Source: CAD feature listing. Evaluate the final solid. Frame: model axes, mm. Give positions to 0.01 mm unless a question says otherwise; leave off trailing zeros. Order: outer loops, then holes, each group sorted by start corner. A loop starts at its lowest first (then second) coordinate and runs counter-clockwise, first axis right, second up. Notation, with made-up numbers: M 36,7.5 L 63,7.5 A10 cw 63,24.5 Z; hole C -7,45 d7. An arc over 180 degrees is marked long. Return JSON: item names as keys, results as strings.
from build123d import *

# Parameters (mm, degrees)
F0_W     = 57.15
F0_H     = 38.1
F1_DEPTH = 25.4
F3_DEPTH = 25.4
F5_DEPTH = 25.4


with BuildPart() as f1:
    # F0 (on Front) → F1 (new body)
    with BuildSketch(Plane.XZ):
        with Locations((28.575, 19.05)):
            Rectangle(F0_W, F0_H)
    extrude(amount=F1_DEPTH)

    # F2 (on face) → F3 (cut)
    with BuildSketch(Plane.XZ.offset(25.4)):
        with BuildLine():
            Line((57.15, 38.1), (38.1, 38.1))
            ThreePointArc((38.1, 38.1), (42.301432, 23.251432), (57.15, 19.05))
            Line((57.15, 19.05), (57.15, 38.1))
        make_face()
    extrude(amount=-F3_DEPTH, mode=Mode.SUBTRACT)

    # F4 (on face) → F5 (cut)
    with BuildSketch(Plane.XZ.offset(25.4)):
        with BuildLine():
            Line((0, 38.1), (0, 34.175124))
            ThreePointArc((0, 34.175124), (1.409017, 36.575001), (3.736917, 38.1))
            Line((3.736917, 38.1), (0, 38.1))
        make_face()
    extrude(amount=-F5_DEPTH, mode=Mode.SUBTRACT)


solid = f1.part
1. Draft query along Z for faces 1 (the face through (28, -13, 0)), 2 (the face through (42.143, -12.878, 23.412)), 3 (the face through (0, -13, 17)). Return one class per face: pulls with the +Z half, pulls with the -Z half, needs draft (parallel to the pull), parting line crosses it, or undercut.
Evaluation:
{"face 1": "pulls with the -Z half", "face 2": "undercut", "face 3": "needs draft"}
2. First-contact query: pin 1 (5 mm diameter, centred on x = 20.5, z = 6.5, fed in from +Y). Flat tip, straight axial feed; report the tip coordinate or a pass-through.
Evaluation:
{"pin 1": "stops at y = 0"}
3. Section query C-C (z = 33). Return loops of the section in (x, y), then the cut area to 3 significant figures.
Evaluation:
{"outline": "M 0,-25.4 L 37.73,-25.4 L 37.73,0 L 0,0 Z", "area": "958 mm^2"}
4. Ray query, probe 1 along X at (y, z) = (-5.75, 33); probe 2 along X at (y, z) = (-17.75, 24); probe 3 along Z at (x, y) = (3, -12). Return the intervals inside material, ascending.
Evaluation:
{"probe 1": "x = 0 to 37.73", "probe 2": "x = 0 to 41.6", "probe 3": "z = 0 to 37.77"}
5. Section query B-B (x = 52). Return loops of the section in (y, z).
Evaluation:
{"outline": "M -25.4,0 L 0,0 L 0,18.69 L -25.4,18.69 Z"}
6. Section query A-A (y = -11). Return loops of the section in (x, z).
Evaluation:
{"outline": "M 0,0 L 57.15,0 L 57.15,19.05 A15.82 cw 38.1,38.1 L 3.74,38.1 A6.1 ccw 0,34.18 Z"}
